from build123d import *

# Parameters (mm, degrees)
SKETCH1_R           = 10
SKETCH1_R_2         = 3
BOSS_EXTRUDE1_DEPTH = 4.8
FILLET1_R           = 0.5
FILLET2_R           = 0.1


with BuildPart() as part:
    # Sketch1 → Boss-Extrude1 (new body)
    with BuildSketch(Plane.XY):
        Circle(SKETCH1_R)
        Circle(SKETCH1_R_2, mode=Mode.SUBTRACT)
    extrude(amount=BOSS_EXTRUDE1_DEPTH)

    # Sketch2 → Cut-Revolve1 (revolve, cut)
    with BuildSketch(Plane(origin=(0, 0, 0), x_dir=(1, 0, 0), z_dir=(0, 1, 0)), mode=Mode.PRIVATE) as cut_revolve1_sk:
        with BuildLine():
            Line((-8.5, -1), (-8.5, -1.8))
            ThreePointArc((-8.5, -1.8), (-8.207106781, -2.507106781), (-7.5, -2.8))
            Line((-7.5, -2.8), (-4, -2.8))
            Line((-4, -2.8), (-4, -2.6))
            Line((-4, -2.6), (-3, -2.6))
            Line((-3, -2.6), (-3, 0))
            Line((-3, 0), (-8.5, 0))
            Line((-8.5, 0), (-9.5, 0))
            ThreePointArc((-9.5, 0), (-8.792893219, -0.292893219), (-8.5, -1))
        make_face()
    revolve(cut_revolve1_sk.sketch.rotate(Axis((0, 0, 0), (0, 0, -1)), 180), axis=Axis((0, 0, 0), (0, 0, -1)), mode=Mode.SUBTRACT)

    # Fillet1
    fillet1_edges = [part.edges().sort_by_distance(p)[0] for p in [
        (-10, 0, 4.8),
    ]]
    fillet(fillet1_edges, radius=FILLET1_R)

    # Fillet2
    fillet2_edges = [part.edges().sort_by_distance(p)[0] for p in [
        (-10, 0, 0),
    ]]
    fillet(fillet2_edges, radius=FILLET2_R)


solid = part.part
The model under review builds one solid part; all positions refer to its coordinate system, in mm. A direction names the side the tool comes from. Coordinates: 2 decimals unless noted, no trailing zeros. Order: outer loops, then holes, each group sorted by start corner. A loop starts at its lowest first (then second) coordinate and runs counter-clockwise, first axis right, second up. Notation, with made-up numbers: (60.5, 30.25) -> (76.5, 30.25) arc R19 cw to (76.5, 56.25) -> close; hole circle Ø6 at (53.25, -9). An arc over 180 degrees is marked (long way). Answer in a Markdown table with one row per item.
(1) Wall thickness on line 1 along Y through (x, z) = (0, 3.9); line 2 along Y through (x, z) = (0, 1.3); line 3 along Z through (x, y) = (-5, -4): over which ranges is each line inside the solid? List them lowest first.
Answers:
| item | result |
|---|---|
| line 1 | -10 to -3, 3 to 10 |
| line 2 | -10 to -8.5, 8.5 to 10 |
| line 3 | 2.8 to 4.8 |
(2) Consider section D-D (z = 3.1). Write out the cut boundary in (x, y), plus the area to 3 significant figures.
Answers:
| item | result |
|---|---|
| outline | circle Ø20 at (0, 0); hole circle Ø6 at (0, 0) |
| area | 286 mm² |
(3) Consider section C-C (z = 1.5). Write out the cut boundary in (x, y).
Answers:
| item | result |
|---|---|
| outline | circle Ø20 at (0, 0); hole circle Ø17 at (0, 0) |
(4) Insertion check: pin 1 (3.5 mm diameter, centred on x = 0, y = 0, fed in from +Z); pin 2 (12 mm diameter, centred on x = -1, y = 0, fed in from -Z); pin 3 (1.5 mm diameter, centred on x = -1, z = 0.5, fed in from +Y); pin 4 (1 mm diameter, centred on y = 1, z = 0.5, fed in from -X). Each pin has a flat end and moves straight along its axis. Give the tip position at first contact, or say it passes through.
Answers:
| item | result |
|---|---|
| pin 1 | through |
| pin 2 | z = 2.6 |
| pin 3 | y = 10 |
| pin 4 | x = -9.99 |
(5) Consider section A-A (y = 0). Write out the cut boundary in (x, z), plus the area to 3 significant figures.
Answers:
| item | result |
|---|---|
| outline | (-10, 0.1) arc R0.1 ccw to (-9.9, 0) -> (-9.5, 0) arc R1 ccw to (-8.5, 1) -> (-8.5, 1.8) arc R1 cw to (-7.5, 2.8) -> (-4, 2.8) -> (-4, 2.6) -> (-3, 2.6) -> (-3, 4.8) -> (-9.5, 4.8) arc R0.5 ccw to (-10, 4.3) -> close; (3, 2.6) -> (4, 2.6) -> (4, 2.8) -> (7.5, 2.8) arc R1 cw to (8.5, 1.8) -> (8.5, 1) arc R1 ccw to (9.5, 0) -> (9.9, 0) arc R0.1 ccw to (10, 0.1) -> (10, 4.3) arc R0.5 ccw to (9.5, 4.8) -> (3, 4.8) -> close |
| area | 36.7 mm² |
(6) Machinability: for faces 1 (the flat face through (1, -3, 2.6)), 2 (the cylindrical face through (-3, 0, 4)), which of the approach directions +Z, -Z, +X, -X, +Y, -Y give a long, thin tool a straight path to every point of the face, cutting with its end or side? Answer none if there is none.
Answers:
| item | result |
|---|---|
| face 1 | -Z |
| face 2 | +Z, -Z |
